Build history of the part. All positions in model axes, mm. Face numbers are marked on the shaded views. A direction names the side the tool comes from. Round coordinates to 2 decimals unless told otherwise and drop trailing zeros. Write each loop counter-clockwise with the first axis right and the second up, starting at its lowest first coordinate (ties: lowest second). Pieces come first, ordered by that corner, then holes. Notation, with made-up numbers: (47.25, 46) -> (55.25, 46) arc R11 ccw to (55.25, 52) -> close; hole circle Ø10 at (-18.5, 72). An arc over 180 degrees is marked (long way). One line per question, with ' | ' between items.
Autodesk Fusion 360 part; units mm, degrees
sketch "Sketch1" plane through (0, 0, 0) normal (0, 0, 1) x (1, 0, 0)
  line L0 (-65, 50) -> (42, 50)
  line L1 (42, 50) -> (42, -17)
  line L2 (42, -17) -> (-65, -17)
  line L3 (-65, -17) -> (-65, 50)
  line L4 (-64, 49) -> (41, 49)
  line L5 (41, 49) -> (41, -16)
  line L6 (41, -16) -> (-64, -16)
  line L7 (-64, -16) -> (-64, 49)
  line L8 (-70, 55) -> (47, 55)
  line L9 (47, 55) -> (47, -22)
  line L10 (47, -22) -> (-70, -22)
  line L11 (-70, -22) -> (-70, 55)
  circle A0 centre (-67, 52) radius 1.3
  circle A1 centre (-67, -19) radius 1.3
  circle A2 centre (44, -19) radius 1.3
  circle A3 centre (44, 52) radius 1.3
  line L12 (-65, 33) -> (-64, 33)
  line L13 (-64, 33) -> (-64, 22.5)
  line L14 (-64, 22.5) -> (-65, 22.5)
  line L15 (-65, 22.5) -> (-65, 33)
  line L16 (18.5, 47.1) -> (36.3, 47.1)
  line L17 (36.3, 47.1) -> (36.3, 26.1)
  line L18 (36.3, 26.1) -> (18.5, 26.1)
  line L19 (18.5, 26.1) -> (18.5, 47.1)
  line L20 (22.9, 58) -> (31.9, 58)
  line L21 (31.9, 58) -> (31.9, 38)
  line L22 (31.9, 38) -> (22.9, 38)
  line L23 (22.9, 38) -> (22.9, 58)
  dimension "d1" = 107
  dimension "d2" = 67
  dimension "d3" = 105
  dimension "d4" = 65
  dimension "d5" = 1
  dimension "d6" = 1
  dimension "d7" = 117
  dimension "d8" = 77
  dimension "d9" = 5
  dimension "d10" = 5
  dimension "d11" = 2.6
  dimension "d12" = 2.6
  dimension "d13" = 2.6
  dimension "d14" = 2.6
  dimension "d15" = 3
  dimension "d16" = 3
  dimension "d17" = 3
  dimension "d18" = 3
  dimension "d19" = 3
  dimension "d20" = 3
  dimension "d21" = 3
  dimension "d22" = 3
  dimension "d23" = 1
  dimension "d24" = 10.5
  dimension "d25" = 17
  dimension "d26" = 17.8
  dimension "d27" = 21
  dimension "d28" = 1.9
  dimension "d29" = 4.7
  dimension "d30" = 9
  dimension "d31" = 20
  dimension "d32" = 4.4
extrude "Extrude1" add sketch "Sketch1" along normal blind 3 contours L0 L1 L2 L3 L8 L9 L10 L11 L15 L21 L23 | L0 L3 L4 L7 L12 L23 | L0 L8 L21 L23 | L0 L4 L21 L23 | L0 L1 L2 L3 L4 L5 L6 L7 L14 L21 | L4 L5 L6 L7 L13 L16 L17 L18 L19 L21 L23 | L4 L16 L21 L23 | L16 L17 L18 L19 L21 L22 L23 | L16 L21 L22 L23
extrude "Extrude2" add sketch "Sketch1" along normal blind 5 contours L0 L3 L4 L7 L12 L23 | L0 L4 L21 L23 | L0 L1 L2 L3 L4 L5 L6 L7 L14 L21
extrude "Extrude3" add 1 faces at (6, -16.6667, 5) along direction (0, 0, 1) blind 1
extrude "Extrude4" add 1 faces at (-68.3333, 18.5, 3) along direction (0, 0, 1) blind 13
extrude "Extrude5" cut sketch "Sketch1" along normal blind 12 contours L0 L8 L21 L23
extrude "Extrude6" add sketch "Sketch1" along normal blind 7 contours L0 L8 L21 L23
sketch "Sketch2" plane through (0, 55, 0) normal (0, 1, 0) x (-1, 0, 0)
  line L0 (-31.9, 7) -> (-31.9, 12)
  line L1 (-31.9, 12) -> (-22.9, 12)
  line L2 (-22.9, 12) -> (-22.9, 7)
  line L3 (-22.9, 7) -> (-31.9, 7)
  line L4 (-47, 0) -> (70, 0)
  line L5 (70, 0) -> (70, 16)
  line L6 (70, 16) -> (-47, 16)
  line L7 (-47, 16) -> (-47, 0)
  line L8 (-34.9, 14.5) -> (-19.9, 14.5)
  line L9 (-19.9, 14.5) -> (-19.9, 4.5)
  line L10 (-19.9, 4.5) -> (-34.9, 4.5)
  line L11 (-34.9, 4.5) -> (-34.9, 14.5)
  dimension "d45" = 15
  dimension "d46" = 10
  dimension "d47" = 3
  dimension "d48" = 2.5
extrude "Extrude7" cut sketch "Sketch2" against normal blind 4.5 contours L8 L9 L10 L11
fillet "Fillet1" radius 1 4 edges at (19.9, 52.75, 4.5) (34.9, 52.75, 4.5) (34.9, 52.75, 14.5) (19.9, 52.75, 14.5)
fillet "Fillet2" radius 1 8 edges at (20.1929, 55, 4.7929) (27.4, 55, 4.5) (34.6071, 55, 4.7929) (34.9, 55, 9.5) (34.6071, 55, 14.2071) (27.4, 55, 14.5) (20.1929, 55, 14.2071) (19.9, 55, 9.5)
extrude "Extrude8" add sketch "Sketch1" along normal blind 10 contours A0 | A1 | A2 | A3
fillet "Fillet3" radius 1.5 4 edges at (47, -22, 8) (47, 55, 8) (-70, 55, 8) (-70, -22, 8)
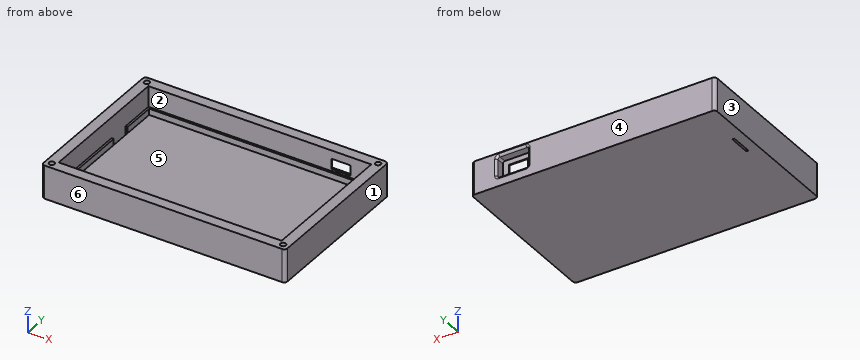
(1) Slice it at C-C (x = 44). Write the cut outline in (y, z), then the cut area to 3 significant figures.
Calculated:
outline: (-22, 0) -> (55, 0) -> (55, 16) -> (53.3, 16) -> (53.3, 10) -> (50.7, 10) -> (50.7, 16) -> (-17.7, 16) -> (-17.7, 10) -> (-20.3, 10) -> (-20.3, 16) -> (-22, 16) -> close | area: 1,200 mm2
(2) Slice it at A-A (y = 52). Write the cut outline in (x, z).
Calculated:
outline: (-70, 0) -> (47, 0) -> (47, 16) -> (45.3, 16) -> (45.3, 10) -> (42.7, 10) -> (42.7, 16) -> (-65.7, 16) -> (-65.7, 10) -> (-68.3, 10) -> (-68.3, 16) -> (-70, 16) -> close; hole (19.9, 5.5) arc R1 ccw to (20.9, 4.5) -> (33.9, 4.5) arc R1 ccw to (34.9, 5.5) -> (34.9, 13.5) arc R1 ccw to (33.9, 14.5) -> (20.9, 14.5) arc R1 ccw to (19.9, 13.5) -> close
(3) 3-axis set-ups, long thin cutter, end or side, ignore diameter. For the marked faces 1 and 2: which of +Z, -Z, +X, -X, +Y, -Y reach the whole face in a straight line?
Calculated:
face 1: +Z, -Z, +X, +Y, -Y | face 2: +Z
(4) Mould opens along Y. For the marked faces 3, 4, 5 and 6 say: pulls with the +Y half, pulls with the -Y half, needs draft (parallel to the pull), parting line crosses it, or undercut.
Calculated:
face 3: needs draft | face 4: pulls with the +Y half | face 5: undercut | face 6: pulls with the -Y half
(5) Slice it at B-B (y = 25.5). Write the cut outline in (x, z).
Calculated:
outline: (-70, 0) -> (-65, 0) -> (-65, 16) -> (-70, 16) -> close; (-64, 0) -> (47, 0) -> (47, 16) -> (42, 16) -> (42, 6) -> (41, 6) -> (41, 3) -> (-64, 3) -> close
(6) Slice it at D-D (y = -3). Write the cut outline in (x, z), then the cut area to 3 significant figures.
Calculated:
outline: (-70, 0) -> (47, 0) -> (47, 16) -> (42, 16) -> (42, 6) -> (41, 6) -> (41, 3) -> (-64, 3) -> (-64, 6) -> (-65, 6) -> (-65, 16) -> (-70, 16) -> close | area: 487 mm2
(7) Drop flat-ended pins along their axis: pin 1 (3 mm diameter, centred on x = 30, z = 11, fed in from +Y); pin 2 (2 mm diameter, centred on x = 44, y = 52, fed in from +Z); pin 3 (4 mm diameter, centred on x = -50.5, y = -11, fed in from +Z). Give the stop position or say it passes through.
Calculated:
pin 1: y = 50.5 | pin 2: z = 10 | pin 3: z = 3
(8) Wall check: line 1 (Y direction, x = 44, z = 13.65); line 2 (X direction, y = 13.5, z = 4); line 3 (X direction, y = 12, z = 11.25). Give the ranges that are in metal, low to high. Write a range as from..to.
Calculated:
line 1: -22..-20.3, -17.7..50.7, 53.3..55 | line 2: -70..-64, 41..47 | line 3: -70..-65, 42..47
